```python
from build123d import *

# Parameters (mm, degrees)
SKETCH1_R           = 30
SKETCH1_R_2         = 15
BOSS_EXTRUDE1_DEPTH = 15
BOSS_EXTRUDE2_DEPTH = 30
SKETCH3_W           = 100
SKETCH3_H           = 200
BOSS_EXTRUDE3_DEPTH = 4
SKETCH4_W           = 20
SKETCH4_H           = 5
CUT_EXTRUDE1_DEPTH  = 4


with BuildPart() as part:
    # Sketch1 → Boss-Extrude1 (new body, symmetric)
    with BuildSketch(Plane.XY):
        Circle(SKETCH1_R)
        Circle(SKETCH1_R_2, mode=Mode.SUBTRACT)
    extrude(amount=BOSS_EXTRUDE1_DEPTH, both=True)

    # Sketch2 → Boss-Extrude2 (add)
    with BuildSketch(Plane.XY.offset(15)):
        with BuildLine():
            Line((14.241500135, 95.50219019), (14.241500135, 360))
            Line((14.241500135, 360), (-14.241500135, 360))
            Line((-14.241500135, 360), (-14.241500135, 95.50219019))
            add(Edge.make_bspline(
                [(-27.670395385, 11.590911061), (-13.495600511, 52.469413615), (-14.241500135, 95.50219019)],
                knots=[0, 0, 0, 1, 1, 1], degree=2))
            ThreePointArc((-27.670395385, 11.590911061), (0, 30), (27.670395385, 11.590911061))
            add(Edge.make_bspline(
                [(27.670395385, 11.590911061), (13.495600511, 52.469413615), (14.241500135, 95.50219019)],
                knots=[0, 0, 0, 1, 1, 1], degree=2))
        make_face()
    extrude(amount=-BOSS_EXTRUDE2_DEPTH)

    # Sketch3 → Boss-Extrude3 (add)
    with BuildSketch(Plane(origin=(0, 360, 0), x_dir=(1, 0, 0), z_dir=(0, 1, 0))):
        Rectangle(SKETCH3_W, SKETCH3_H)
    extrude(amount=-BOSS_EXTRUDE3_DEPTH)

    # Sketch4 → Cut-Extrude1 (cut)
    with BuildSketch(Plane.XZ.offset(-356)):
        with Locations((30, 87.5)):
            Rectangle(SKETCH4_W, SKETCH4_H)
        with Locations((-30, 87.5)):
            Rectangle(SKETCH4_W, SKETCH4_H)
        with Locations((-30, -87.5)):
            Rectangle(SKETCH4_W, SKETCH4_H)
        with Locations((30, -87.5)):
            Rectangle(SKETCH4_W, SKETCH4_H)
        with Locations((-30, 52.5)):
            Rectangle(SKETCH4_W, SKETCH4_H)
        with Locations((30, 52.5)):
            Rectangle(SKETCH4_W, SKETCH4_H)
        with Locations((30, -52.5)):
            Rectangle(SKETCH4_W, SKETCH4_H)
        with Locations((-30, -52.5)):
            Rectangle(SKETCH4_W, SKETCH4_H)
    extrude(amount=-CUT_EXTRUDE1_DEPTH, mode=Mode.SUBTRACT)


solid = part.part
```
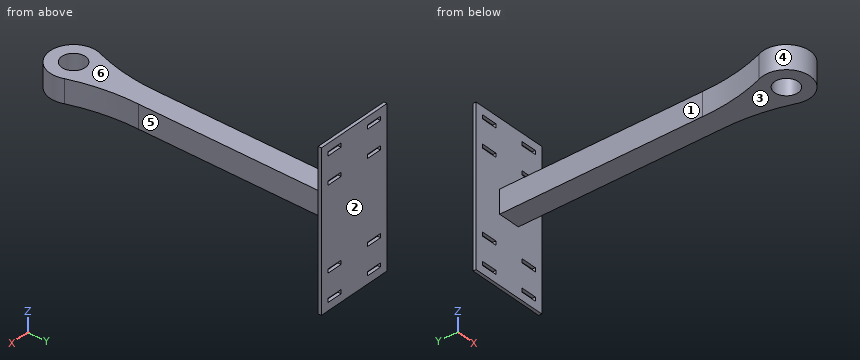
CAD build for the part. Positions are in the model's coordinates, mm. Face numbers are marked on the shaded views. A direction names the side the tool comes from. Coordinates: 2 decimals unless noted, no trailing zeros. Order: outer loops, then holes, each group sorted by start corner. A loop starts at its lowest first (then second) coordinate and runs counter-clockwise, first axis right, second up. Notation, with made-up numbers: (18.25, 15.25) -> (77.25, 15.25) arc R28 ccw to (77.25, 36.25) -> close; hole circle Ø9 at (53, 42.5). An arc over 180 degrees is marked (long way). Use one line per item in the form item = value. Start each with the question number.
1) Band-saw the part on D-D on y = 317. Give the cut face in (x, z), then the cut area to 3 significant figures.
2) Band-saw the part on B-B on y = 0. Give the cut face in (x, z).
3) Tool access for the marked faces 4, 5 and 6: list every direction of +Z, -Z, +X, -X, +Y, -Y with a clear straight run to the whole face (end or side of a thin tool).
4) Drill centre lines: L1, parallel to Y at x = 0, z = -5; L2, parallel to Y at x = -24, z = 80; L3, parallel to X at y = 164, z = -14.5. Where is each one in solid material? Low to high. Write a range as [from, to].
5) Drop flat-ended pins along their axis: pin 1 (5 mm diameter, centred on x = 24.5, z = 66, fed in from -Y); pin 2 (2 mm diameter, centred on y = 206, z = -8, fed in from -X). Give the stop position or say it passes through.
6) Band-saw the part on A-A on x = -34. Give the cut face in (y, z), then the cut area to 3 significant figures.
7) Pull direction Y, two halves, no side cores. Call the marked faces 1, 2 and 3: +Y half, -Y half, draft (parallel to the pull), parting line (faces both ways), or undercut.
8) Band-saw the part on C-C on x = 0. Give the cut face in (y, z).
Entries:
q1.outline = (-14.24, -15) -> (14.24, -15) -> (14.24, 15) -> (-14.24, 15) -> close
q1.area = 854 mm2
q2.outline = (-30, -15) -> (-15, -15) -> (-15, 15) -> (-30, 15) -> close; (15, -15) -> (30, -15) -> (30, 15) -> (15, 15) -> close
q3.face_4 = +Z, -Z
q3.face_5 = +Z, -Z, +X
q3.face_6 = +Z, +X, -X, -Y
q4.L1 = [-30, -15], [15, 360]
q4.L2 = [356, 360]
q4.L3 = [-14.24, 14.24]
q5.pin_1 = 356
q5.pin_2 = -14.24
q6.outline = (356, -100) -> (360, -100) -> (360, -90) -> (356, -90) -> close; (356, -85) -> (360, -85) -> (360, -55) -> (356, -55) -> close; (356, -50) -> (360, -50) -> (360, 50) -> (356, 50) -> close; (356, 55) -> (360, 55) -> (360, 85) -> (356, 85) -> close; (356, 90) -> (360, 90) -> (360, 100) -> (356, 100) -> close
q6.area = 720 mm2
q7.face_1 = undercut
q7.face_2 = +Y half
q7.face_3 = draft
q8.outline = (-30, -15) -> (-15, -15) -> (-15, 15) -> (-30, 15) -> close; (15, -15) -> (356, -15) -> (356, -100) -> (360, -100) -> (360, 100) -> (356, 100) -> (356, 15) -> (15, 15) -> close
